```python
from build123d import *

# Parameters (mm, degrees)
SKETCH035_R     = 2.475
SKETCH035_R_2   = 3.4
PAD019_DEPTH    = 7
SKETCH036_W     = 11.870498
SKETCH036_H     = 2.853485
SKETCH036_W_2   = 11.727337
SKETCH036_H_2   = 2.709564
PAD020_DEPTH    = 1.8
SKETCH037_R     = 16.1879
POCKET019_DEPTH = 3
SKETCH038_W     = 2.5
SKETCH038_H     = 1.25
POCKET020_DEPTH = 1
FILLET003_R     = 0.4


with BuildPart() as part:
    # Sketch035 (on DatumPlane) → Pad019 (new body)
    with BuildSketch(Plane.YZ.offset(-30)):
        with BuildLine():
            Line((60.863192, -45.726101), (60.863192, -94.755177))
            Line((60.863192, -94.755177), (1.18502, -84.232305))
            ThreePointArc((1.18502, -56.248973), (-10.555381, -70.240639), (1.18502, -84.232305))
            Line((60.863192, -45.726101), (1.18502, -56.248973))
        make_face()
        with Locations((34.863192, -70.240639)):
            Circle(SKETCH035_R, mode=Mode.SUBTRACT)
        with Locations((4.863192, -70.240639)):
            Circle(SKETCH035_R_2, mode=Mode.SUBTRACT)
    extrude(amount=-PAD019_DEPTH)

    # Sketch036 (on Face1 of Pad019) → Pad020 (join)
    with BuildSketch(Plane.ZX.offset(60.863192)):
        with Locations((-84.965439, -35.379314)):
            Rectangle(SKETCH036_W, SKETCH036_H)
        with Locations((-58.534715, -35.418369)):
            Rectangle(SKETCH036_W_2, SKETCH036_H_2)
    extrude(amount=PAD020_DEPTH)

    # Sketch037 (on Face4 of Pad020) → Pocket019 (cut)
    with BuildSketch(Plane(origin=(-37, 0, 0), x_dir=(0, 1, 0), z_dir=(-1, 0, 0))):
        with Locations((4.863192, 70.240639)):
            Circle(SKETCH037_R)
    extrude(amount=-POCKET019_DEPTH, mode=Mode.SUBTRACT)

    # Sketch038 (on Face15 of Pocket019) → Pocket020 (cut)
    with BuildSketch(Plane(origin=(-34, 0, 0), x_dir=(0, 1, 0), z_dir=(-1, 0, 0))):
        with Locations((4.863192, 62.458053)):
            Rectangle(SKETCH038_W, SKETCH038_H)
    extrude(amount=-POCKET020_DEPTH, mode=Mode.SUBTRACT)

    # Fillet003
    fillet003_edges = [part.edges().sort_by_distance(p)[0] for p in [
        (-34.063587, 62.663192, -58.534716),
        (-35.418369, 62.663192, -52.671047),
        (-36.773151, 62.663192, -58.534716),
        (-35.418369, 62.663192, -64.398384),
        (-33.952572, 62.663192, -84.965439),
        (-35.379314, 62.663192, -79.03019),
        (-36.806057, 62.663192, -84.965439),
        (-35.379314, 62.663192, -90.900688),
    ]]
    fillet(fillet003_edges, radius=FILLET003_R)


solid = part.part
```
Model file for the job. Use its own axes, mm. A direction names the side the tool comes from. Give positions to 0.01 mm unless a question says otherwise; leave off trailing zeros. Loops run counter-clockwise (first coordinate to the right, second up) from the corner with the lowest first, then second, coordinate; pieces in that order, holes last. Notation, with made-up numbers: M -32,70.5 L -26,70.5 A29 ccw -26,92.5 Z; hole C -16.5,3.5 d4. An arc over 180 degrees is marked long. Use one line per item in the form item = value.
Item 1: Two-plate mould, pull along Y, no slides. Class faces 1 (the flat face through (-34, 9, -70)), 2 (the cylindrical face through (-33.45, 36.19, -68.15)), 3 (the flat face through (-33.451, 31.442, -89.567)): released by +Y, released by -Y, zero draft, split by the parting line, or undercut.
Filled in:
face_1 = zero draft
face_2 = undercut
face_3 = released by -Y
Item 2: Slice it at B-B on x = -31.5. List the corners of the cut face in (y, z) (3 decimals), and give its area (3 significant figures).
Filled in:
outline = M 1.185,-84.232 L 60.863,-94.755 L 60.863,-45.726 L 1.185,-56.249 A14.208 ccw Z; hole C 4.863,-70.241 d6.8; hole C 34.863,-70.241 d4.95
area = 2,490 mm^2
Item 3: Slice it at D-D on z = -57. List the corners of the cut face in (x, y), and give its area (3 significant figures).
Filled in:
outline = M -37,14.18 L -34,14.18 L -34,-1.5 L -30,-1.5 L -30,60.86 L -34.06,60.86 L -34.06,62.26 A0.4 ccw -34.46,62.66 L -36.37,62.66 A0.4 ccw -36.77,62.26 L -36.77,60.86 L -37,60.86 Z
area = 394 mm^2
Item 4: Which spindle directions (+Z, -Z, +X, -X, +Y, -Y) get a long thin tool onto all of the face, cutting with end or side? Do faces 4 (the flat face through (-33.953, 62, -85)), 5 (the cylindrical face through (-35.52, 21.05, -69.95)), 6 (the flat face through (-34.064, 62, -59)), 7 (the flat face through (-35, 62, -90.901)). Say none if no direction does.
Filled in:
face_4 = +Z, -Z, +X, +Y
face_5 = -X, -Y
face_6 = +Z, +X, +Y
face_7 = -Z, +X, -X, +Y
Item 5: Slice it at C-C on y = 17. List the corners of the cut face in (x, z), and give its area (3 significant figures).
Filled in:
outline = M -37,-87.02 L -30,-87.02 L -30,-53.46 L -37,-53.46 L -37,-59.53 L -34,-59.53 L -34,-80.95 L -37,-80.95 Z
area = 171 mm^2
Item 6: Slice it at A-A on y = 7. List the corners of the cut face in (x, z), and give its area (3 significant figures).
Filled in:
outline = M -34,-85.26 L -30,-85.26 L -30,-72.89 L -34,-72.89 Z; M -34,-67.6 L -30,-67.6 L -30,-55.22 L -34,-55.22 Z
area = 99.0 mm^2
Item 7: Drill centre lines: L1, parallel to X at y = 10.5, z = -63; L2, parallel to Z at x = -36.5, y = 12; L3, parallel to Z at x = -35.25, y = 33.5. Where is each one in solid material? Low to high.
Filled in:
L1 = -34 to -30
L2 = -86.14 to -84.77, -55.71 to -54.34
L3 = -89.93 to -72.31, -68.17 to -50.55
Item 8: Flat gauge pins, fed straight in: pin 1 Ø1.1 at (x, y) = (-36, 61) entering from +Z; pin 2 Ø3 at (x, y) = (-35.5, 48.5) entering from -Z; pin 3 Ø4 at (y, z) = (4.86, -70.24) entering from -X; pin 4 Ø1.1 at (x, y) = (-36, 61.5) entering from -Z. Where does each tip first touch, or does it go through?
Filled in:
pin_1 = -45.73
pin_2 = -92.84
pin_3 = through
pin_4 = -90.9
